Autodesk Inventor part; units mm, degrees
ref_plane "YZ Plane" through (0, 0, 0) normal (1, 0, 0) x (0, 1, 0)
ref_plane "XZ Plane" through (0, 0, 0) normal (0, 1, 0) x (-1, 0, 0)
ref_plane "XY Plane" through (0, 0, 0) normal (0, 0, 1) x (1, 0, 0)
sketch "Skizze1" plane through (0, 0, 0) normal (0, 0, 1) x (1, 0, 0)
  circle A0 centre (0, 0) radius 22.035
  dimension "d0" = 44.07
extrude "Extrusion1" add sketch "Skizze1" along normal blind 1.5
sketch "Skizze2" plane through (0, 0, 1.5) normal (0, 0, 1) x (1, 0, 0)
  circle A0 centre (0, 0) radius 19.5
  dimension "d3" = 39
extrude "Extrusion2" add sketch "Skizze2" along normal blind 8
sketch "Skizze3" plane through (0, 0, 9.5) normal (0, 0, 1) x (1, 0, 0)
  circle A0 centre (0, 0) radius 9.75
  dimension "d6" = 19.5
extrude "Extrusion3" add sketch "Skizze3" along normal blind 4.2
sketch "Skizze4" plane through (0, 0, 13.7) normal (0, 0, 1) x (1, 0, 0)
  circle A0 centre (0, 0) radius 19.5
  dimension "d12" = 39
extrude "Extrusion4" add sketch "Skizze4" along normal blind 6
fillet "Rundung1" radius 1.5 1 edges at (-19.5, 0, 19.7)
sketch "Skizze5" plane through (0, 0, 19.7) normal (0, 0, 1) x (1, 0, 0)
  circle A0 centre (0, 0) radius 3.25
  dimension "d13" = 6.5
extrude "Extrusion5" cut sketch "Skizze5" against normal blind 100
Input: part model. Units: mm. Frame: model coordinates. A direction names the side the tool comes from. Give positions to 0.01 mm unless a question says otherwise; leave off trailing zeros. Order: outer loops, then holes, each group sorted by start corner. A loop starts at its lowest first (then second) coordinate and runs counter-clockwise, first axis right, second up.
Q1. Ray query, probe 1 along Z at (x, y) = (8.5, -7); probe 2 along Y at (x, z) = (0, 7.75); probe 3 along Y at (x, z) = (0, 13.25). Return the intervals inside material, ascending.
Checked values:
probe 1: z = 0 to 9.5, 13.7 to 19.7
probe 2: y = -19.5 to -3.25, 3.25 to 19.5
probe 3: y = -9.75 to -3.25, 3.25 to 9.75
Q2. Section C-C on z = 13. Output: boundary loops of the cut face in (x, y), and give its area (3 significant figures).
Checked values:
outline: circle Ø19.5 at (0, 0); hole circle Ø6.5 at (0, 0)
area: 265 mm2
Q3. Contact query for flat-ended pins moving along their axis: pin 1 Ø10 at (x, z) = (-5.5, 4.5) entering from +Y; pin 2 Ø2 at (x, z) = (-10, 3.5) entering from -Y; pin 3 Ø5 at (y, z) = (-13.5, 6.5) entering from +X. Output: stop coordinate, or through.
Checked values:
pin 1: stops at y = 21.98
pin 2: stops at y = -17.3
pin 3: stops at x = 16.1
Q4. Section A-A on x = 0. Output: boundary loops of the cut face in (y, z) (3 decimals), and give its area (3 significant figures).
Checked values:
outline: (-22.035, 0) - (-3.25, 0) - (-3.25, 19.7) - (-18, 19.7) arc R1.5 ccw to (-19.5, 18.2) - (-19.5, 13.7) - (-9.75, 13.7) - (-9.75, 9.5) - (-19.5, 9.5) - (-19.5, 1.5) - (-22.035, 1.5) - close; (3.25, 0) - (22.035, 0) - (22.035, 1.5) - (19.5, 1.5) - (19.5, 9.5) - (9.75, 9.5) - (9.75, 13.7) - (19.5, 13.7) - (19.5, 18.2) arc R1.5 ccw to (18, 19.7) - (3.25, 19.7) - close
area: 565 mm2
Q5. Draft query along X for faces 4 (the flat face through (0, -4, 19.7)), 5 (the cylindrical face through (-2.579, -1.978, 9.988)), 6 (the cylindrical face through (-2.539, -19.334, 5.444)). Return one class per face: +X half, -X half, draft (parallel to the pull), parting line (faces both ways), or undercut.
Checked values:
face 4: draft
face 5: undercut
face 6: parting line
Q6. Section B-B on z = 3.25. Output: boundary loops of the cut face in (x, y), and give its area (3 significant figures).
Checked values:
outline: circle Ø39 at (0, 0); hole circle Ø6.5 at (0, 0)
area: 1,160 mm2
Q7. Set-up query: faces 1 (the cylindrical face through (-1.269, -9.667, 11.571)), 2 (the cylindrical face through (-17.486, 13.408, 0.74)), 3 (the flat face through (8, -18, 1.5)). Return all of +Z, -Z, +X, -X, +Y, -Y with unobstructed straight access to the full face (end or side cutting, diameter ignored); none if empty.
Checked values:
face 1: none
face 2: +Z, -Z
face 3: +Z
